```python
from build123d import *

# Parameters (mm, degrees)
SKETCH3_R          = 5
CUT_EXTRUDE1_DEPTH = 67.708320321


with BuildPart() as part:
    # Sketch2 → Revolve1 (revolve)
    with BuildSketch(Plane.XY, mode=Mode.PRIVATE) as revolve1_sk:
        Polygon((0, 15), (20, 15), (20, 30), (10, 30), (10, 45), (0, 45), align=None)
    revolve(revolve1_sk.sketch.rotate(Axis((0, 0, 0), (1, 0, 0)), 90), axis=Axis((0, 0, 0), (1, 0, 0)))

    # Sketch3 → Cut-Extrude1 (cut, through all)
    with BuildSketch(Plane.ZY):
        with Locations((0, 37.5)):
            Circle(SKETCH3_R)
        with Locations((26.516504294, 26.516504294)):
            Circle(SKETCH3_R)
        with Locations((37.5, 0)):
            Circle(SKETCH3_R)
        with Locations((26.516504294, -26.516504294)):
            Circle(SKETCH3_R)
        with Locations((0, -37.5)):
            Circle(SKETCH3_R)
        with Locations((-26.516504294, -26.516504294)):
            Circle(SKETCH3_R)
        with Locations((-37.5, 0)):
            Circle(SKETCH3_R)
        with Locations((-26.516504294, 26.516504294)):
            Circle(SKETCH3_R)
    extrude(amount=-CUT_EXTRUDE1_DEPTH, mode=Mode.SUBTRACT)


solid = part.part
```
The listing builds one solid part. Answer for the finished solid, in the listing's coordinates (mm). A direction names the side the tool comes from. Coordinates: 2 decimals unless noted, no trailing zeros. Loops run counter-clockwise (first coordinate to the right, second up) from the corner with the lowest first, then second, coordinate; pieces in that order, holes last. Notation, with made-up numbers: M 88,47.5 L 136,47.5 A28 ccw 136,71.5 Z; hole C 16.25,74 d10. An arc over 180 degrees is marked long. Answer as a JSON object with one key per item and string values. Group by question number.
Item 1: Section C-C (z = -37.5) is taken. Write down the section's boundary in (x, y).
Item 2: Section D-D (z = -27.5) is taken. Write down the section's boundary in (x, y).
Item 3: Determine the mould class of faces 3 (the face through (0, -11, -11)), 4 (the face through (14.93, -25.296, 16.128)), 5 (the face through (4.93, 0.22, 32.505)) for opening direction Z: +Z half, -Z half, draft (parallel to the pull), parting line (faces both ways), or undercut.
Item 4: Consider L1, parallel to Y at x = 8, z = -0.5; L2, parallel to Z at x = 4, y = -24; L3, parallel to Y at x = 7.75, z = -33.5. Determine where each line is inside the solid, lowest interval first.
Item 5: Which of the six approach directions +Z, -Z, +X, -X, +Y, -Y give full straight-line access (tool end or side, diameter ignored) to faces 1 (the face through (4.93, -33.284, 2.688)), 2 (the face through (10, -31, 1))?
Item 6: Section A-A (z = 0) is taken. Write down the section's boundary in (x, y).
Item 7: Each of these flat-tipped pins is pushed along its axis until it touches: P1, Ø8, axis at x = 13, y = 2, coming from the -Z side; P2, Ø6, axis at y = -37.5, z = 0, coming from the +X side; P3, Ø5, axis at x = 11, z = 34, coming from the +Y side; P4, Ø5, axis at x = 15.5, z = -6.5, coming from the -Y side. Where does it stop, or does it pass through?
Solved:
{
 "1": {"outline": "M 0,-24.87 L 10,-24.87 L 10,-5 L 0,-5 Z; M 0,5 L 10,5 L 10,24.87 L 0,24.87 Z"},
 "2": {"outline": "M 0,-35.62 L 10,-35.62 L 10,-31.42 L 0,-31.42 Z; M 0,-21.61 L 10,-21.61 L 10,-11.99 L 20,-11.99 L 20,11.99 L 10,11.99 L 10,21.61 L 0,21.61 Z; M 0,31.42 L 10,31.42 L 10,35.62 L 0,35.62 Z"},
 "3": {"face 3": "draft", "face 4": "parting line", "face 5": "undercut"},
 "4": {"L1": "y = -45 to -42.47, -32.53 to -14.99, 14.99 to 32.53, 42.47 to 45", "L2": "z = -38.07 to -30.84, -22.2 to 22.2, 30.84 to 38.07", "L3": "y = -30.05 to -3, 3 to 30.05"},
 "5": {"face 1": "+X, -X", "face 2": "+X"},
 "6": {"outline": "M 0,-45 L 10,-45 L 10,-42.5 L 0,-42.5 Z; M 0,-32.5 L 10,-32.5 L 10,-30 L 20,-30 L 20,-15 L 0,-15 Z; M 0,15 L 20,15 L 20,30 L 10,30 L 10,32.5 L 0,32.5 Z; M 0,42.5 L 10,42.5 L 10,45 L 0,45 Z"},
 "7": {"P1": "stops at z = -45", "P2": "passes through", "P3": "stops at y = 31.93", "P4": "stops at y = -29.73"}
}
